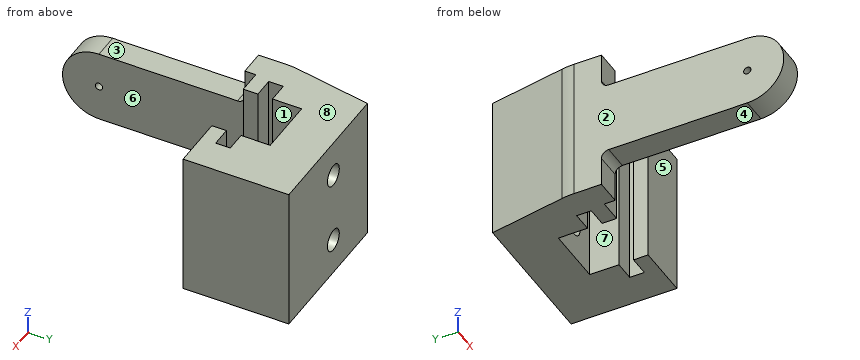
```python
from build123d import *

# Parameters (mm, degrees)
SKETCH1_W           = 22
SKETCH1_H           = 16
BOSS_EXTRUDE1_DEPTH = 20
CHAMFER1_SIZE       = 2
CHAMFER1_SIZE2      = 11.342563639
CUT_EXTRUDE1_DEPTH  = 20
FILLET1_R           = 10
SKETCH3_W           = 3.5
SKETCH3_H           = 10
BOSS_EXTRUDE2_DEPTH = 20
FILLET2_R           = 1
BOSS_EXTRUDE3_DEPTH = 3.5
SKETCH8_R           = 0.5
CUT_EXTRUDE2_DEPTH  = 3.5
SKETCH9_R           = 1.5
CUT_EXTRUDE3_DEPTH  = 6.5


with BuildPart() as part:
    # Sketch1 → Boss-Extrude1 (new body)
    with BuildSketch(Plane.XY):
        with Locations((11, -8)):
            Rectangle(SKETCH1_W, SKETCH1_H)
    extrude(amount=BOSS_EXTRUDE1_DEPTH)

    # Chamfer1
    chamfer1_edges = [part.edges().sort_by_distance(p)[0] for p in [
        (0, 0, 10),
    ]]
    chamfer1_side = [part.faces().sort_by_distance(p)[0] for p in [
        (11, 0, 10),
    ]]
    chamfer(chamfer1_edges, length=CHAMFER1_SIZE, length2=CHAMFER1_SIZE2, reference=chamfer1_side[0])

    # Sketch2 → Cut-Extrude1 (cut)
    with BuildSketch(Plane.XY.offset(20)):
        Polygon((3.5, -16), (3.5, -14.5), (6.67, -14.5), (6.67, -12.5), (3.92, -12.5), (3.92, -10.5), (6.67, -10.5), (6.67, -6.5), (14.67, -6.5), (14.67, -10.5), (17.42, -10.5), (17.42, -12.5), (14.67, -12.5), (14.67, -14.5), (22, -14.5), (22, -16), align=None)
    extrude(amount=-CUT_EXTRUDE1_DEPTH, mode=Mode.SUBTRACT)

    # Fillet1
    fillet1_edges = [part.edges().sort_by_distance(p)[0] for p in [
        (0, -11.342563639, 10),
    ]]
    fillet(fillet1_edges, radius=FILLET1_R)

    # Sketch3 → Boss-Extrude2 (add)
    with BuildSketch(Plane.XZ.offset(16)):
        with Locations((1.75, 10)):
            Rectangle(SKETCH3_W, SKETCH3_H)
    extrude(amount=BOSS_EXTRUDE2_DEPTH)

    # Fillet2
    fillet2_edges = [part.edges().sort_by_distance(p)[0] for p in [
        (1.75, -16, 5),
        (1.75, -16, 15),
    ]]
    fillet(fillet2_edges, radius=FILLET2_R)

    # Sketch7 → Boss-Extrude3 (add)
    with BuildSketch(Plane.ZY):
        with BuildLine():
            Line((15, -36), (5, -36))
            ThreePointArc((5, -36), (10, -41), (15, -36))
        make_face()
    extrude(amount=-BOSS_EXTRUDE3_DEPTH)

    # Sketch8 → Cut-Extrude2 (cut)
    with BuildSketch(Plane.ZY):
        with Locations((10, -36)):
            Circle(SKETCH8_R)
    extrude(amount=-CUT_EXTRUDE2_DEPTH, mode=Mode.SUBTRACT)

    # Sketch9 → Cut-Extrude3 (cut)
    with BuildSketch(Plane.XZ.offset(6.5)):
        with Locations((10.67, 15)):
            Circle(SKETCH9_R)
        with Locations((10.67, 5)):
            Circle(SKETCH9_R)
    extrude(amount=-CUT_EXTRUDE3_DEPTH, mode=Mode.SUBTRACT)


solid = part.part
```
The model under review builds one solid part; all positions refer to its coordinate system, in mm. Face numbers are marked on the shaded views. A direction names the side the tool comes from. Round coordinates to 2 decimals unless told otherwise and drop trailing zeros. Write each loop counter-clockwise with the first axis right and the second up, starting at its lowest first coordinate (ties: lowest second). Pieces come first, ordered by that corner, then holes.
(1) We need section A-A on z = 10. Give the boundary of the cut face in (x, y), and give its area (3 significant figures).
(2) We need section C-C on x = 10.67. Give the boundary of the cut face in (y, z), and give its area (3 significant figures).
(3) We need section D-D on y = -8.5. Give the boundary of the cut face in (x, z).
(4) We need section B-B on x = 2.5. Give the boundary of the cut face in (y, z), and give its area (3 significant figures).
(5) Mouldability with a two-part tool opening along X and no side actions: class the marked faces 6, 7 and 8 as +X half, -X half, draft (parallel to the pull), parting line (faces both ways), or undercut.
(6) Insertion check: pin 1 (1.8 mm diameter, centred on x = 1, z = 18, fed in from -Y); pin 2 (10 mm diameter, centred on x = 6, y = -24.5, fed in from -Z); pin 3 (0.8 mm diameter, centred on x = 5, z = 14.5, fed in from -Y); pin 4 (4 mm diameter, centred on x = 6, y = -24.5, fed in from -Z). Each pin has a flat end and moves straight along its axis. Give the tip position at first contact, or say it passes through.
(7) Wall thickness on L1, parallel to Z at x = 10.67, y = -2.75; L2, parallel to Z at x = 1.35, y = -36; L3, parallel to Y at x = 14.75, z = 5.25: over which ranges is each line inside the solid? List them lowest first.
(8) Machinability: for the marked faces 1, 2, 3, 4 and 5, which of the approach directions +Z, -Z, +X, -X, +Y, -Y give a long, thin tool a straight path to every point of the face, cutting with its end or side? Answer none if there is none.
Findings below:
1. outline: (0, -41) - (3.5, -41) - (3.5, -36.5) - (0, -36.5) - close; (0, -35.5) - (3.5, -35.5) - (3.5, -14.5) - (6.67, -14.5) - (6.67, -12.5) - (3.92, -12.5) - (3.92, -10.5) - (6.67, -10.5) - (6.67, -6.5) - (14.67, -6.5) - (14.67, -10.5) - (17.42, -10.5) - (17.42, -12.5) - (14.67, -12.5) - (14.67, -14.5) - (22, -14.5) - (22, 0) - (2, 0) - (0.15, -10.48) arc R10 ccw to (0, -12.22) - close
1. area: 322 mm2
2. outline: (-6.5, 0) - (0, 0) - (0, 3.5) - (-6.5, 3.5) - close; (-6.5, 6.5) - (0, 6.5) - (0, 13.5) - (-6.5, 13.5) - close; (-6.5, 16.5) - (0, 16.5) - (0, 20) - (-6.5, 20) - close
2. area: 91.0 mm2
3. outline: (0.5, 0) - (6.67, 0) - (6.67, 20) - (0.5, 20) - close; (14.67, 0) - (22, 0) - (22, 20) - (14.67, 20) - close
4. outline: (-36, 5) - (-17, 5) arc R1 cw to (-16, 4) - (-16, 0) - (0, 0) - (0, 20) - (-16, 20) - (-16, 16) arc R1 cw to (-17, 15) - (-36, 15) arc R5 ccw to start; hole circle Ø1 at (-36, 10)
4. area: 559 mm2
5. face 6: +X half
5. face 7: undercut
5. face 8: draft
6. pin 1: stops at y = -16
6. pin 2: stops at z = 5
6. pin 3: stops at y = -14.5
6. pin 4: passes through
7. L1: z = 0 to 3.5, 6.5 to 13.5, 16.5 to 20
7. L2: z = 5 to 9.5, 10.5 to 15
7. L3: y = -14.5 to -12.5, -10.5 to 0
8. face 1: +Z, -Z, -Y
8. face 2: +Z, -Z, -X, +Y, -Y
8. face 3: +Z, +X, -X, -Y
8. face 4: -Z, +X, -X, -Y
8. face 5: +Z, -Z, +X, -Y
